```python
from build123d import *

# Parameters (mm, degrees)
SKETCH1_W           = 12.5
SKETCH1_H           = 4
SKETCH2_W           = 6
SKETCH2_H           = 2
SKETCH2_W_2         = 1.5
SKETCH2_H_2         = 1.5
SKETCH3_R           = 3.15
BOSS_EXTRUDE1_DEPTH = 1.3
SKETCH4_R           = 1.5
BOSS_EXTRUDE2_DEPTH = 4
CIRPATTERN1_COUNT   = 4
CHAMFER1_SIZE       = 1.3
CHAMFER1_SIZE_2     = 0.113735263


with BuildPart() as part:
    # Sketch1 → Revolve1 (revolve)
    with BuildSketch(Plane.XY, mode=Mode.PRIVATE) as revolve1_sk:
        with Locations((13.75, 2)):
            Rectangle(SKETCH1_W, SKETCH1_H)
    revolve(revolve1_sk.sketch.rotate(Axis((0, -5.176379432, 0), (0, 1, 0)), 90), axis=Axis((0, -5.176379432, 0), (0, 1, 0)))

    # Sketch2 → Cut-Revolve1 (revolve, cut)
    with BuildSketch(Plane.XY, mode=Mode.PRIVATE) as cut_revolve1_sk:
        with Locations((17, 1)):
            Rectangle(SKETCH2_W, SKETCH2_H)
        with Locations((8.25, 0.75)):
            Rectangle(SKETCH2_W_2, SKETCH2_H_2)
    revolve(cut_revolve1_sk.sketch.rotate(Axis((0, -1.233398275, 0), (0, 1, 0)), 90), axis=Axis((0, -1.233398275, 0), (0, 1, 0)), mode=Mode.SUBTRACT)

    # Sketch3 → Boss-Extrude1 (add)
    with BuildSketch(Plane(origin=(0, 4, 0), x_dir=(1, 0, 0), z_dir=(0, 1, 0))):
        with Locations(Location((17, 0, 0), (0, 0, 19.305796893))):
            Circle(SKETCH3_R)
    boss_extrude1 = extrude(amount=BOSS_EXTRUDE1_DEPTH)

    # Sketch4 → Boss-Extrude2 (add)
    with BuildSketch(Plane.XZ.offset(-2)):
        with Locations(Location((17, 0, 0), (0, 0, 90))):
            Circle(SKETCH4_R)
    boss_extrude2 = extrude(amount=BOSS_EXTRUDE2_DEPTH)

    # CirPattern1: Boss-Extrude1, Boss-Extrude2 ×4 about axis
    cirpattern1_axis = Axis((0, 0, 0), (0, 1, 0))
    add([boss_extrude1.rotate(cirpattern1_axis, i * 360 / CIRPATTERN1_COUNT) for i in range(1, CIRPATTERN1_COUNT)])
    add([boss_extrude2.rotate(cirpattern1_axis, i * 360 / CIRPATTERN1_COUNT) for i in range(1, CIRPATTERN1_COUNT)])

    # Chamfer1
    # the kernel refuses this chamfer: 1.3, 0.113735263 mm, written as the material it takes off along each edge
    with BuildSketch(Plane(origin=(17, 5.3, 0), x_dir=(0.9437675070022826, 0, -0.3306098799592901), z_dir=(0.3306098799592901, 0, 0.9437675070022826))) as chamfer1_piece_1_section:
        Polygon((3.15, -CHAMFER1_SIZE), (3.15 - CHAMFER1_SIZE_2 * 0.99999999634, 0), (3.15, 0), align=None)
    chamfer1_piece_1 = revolve(axis=Axis((17, 5.3, 0), (0, 1, 0)), mode=Mode.PRIVATE)
    chamfer1_piece_1 = split(chamfer1_piece_1, bisect_by=Plane(origin=(14.070685383, 4, 1.026164121), z_dir=(0, 1, 0)), keep=Keep.TOP, mode=Mode.PRIVATE)
    add(chamfer1_piece_1, mode=Mode.SUBTRACT)
    with BuildSketch(Plane(origin=(0, 5.3, 17), x_dir=(0.3306098799592899, 0, 0.9437675070022828), z_dir=(-0.9437675070022828, 0, 0.3306098799592899))) as chamfer1_piece_2_section:
        Polygon((3.15, -CHAMFER1_SIZE), (3.15 - CHAMFER1_SIZE_2 * 0.99999999634, 0), (3.15, 0), align=None)
    chamfer1_piece_2 = revolve(axis=Axis((0, 5.3, 17), (0, 1, 0)), mode=Mode.PRIVATE)
    chamfer1_piece_2 = split(chamfer1_piece_2, bisect_by=Plane(origin=(-1.026164121, 4, 14.070685383), z_dir=(0, 1, 0)), keep=Keep.TOP, mode=Mode.PRIVATE)
    add(chamfer1_piece_2, mode=Mode.SUBTRACT)
    with BuildSketch(Plane(origin=(-17, 5.3, 0), x_dir=(-0.9437675070022828, 0, 0.33060987995929), z_dir=(-0.33060987995929, 0, -0.9437675070022828))) as chamfer1_piece_3_section:
        Polygon((3.15, -CHAMFER1_SIZE), (3.15 - CHAMFER1_SIZE_2 * 0.99999999634, 0), (3.15, 0), align=None)
    chamfer1_piece_3 = revolve(axis=Axis((-17, 5.3, 0), (0, 1, 0)), mode=Mode.PRIVATE)
    chamfer1_piece_3 = split(chamfer1_piece_3, bisect_by=Plane(origin=(-14.070685383, 4, -1.026164121), z_dir=(0, 1, 0)), keep=Keep.TOP, mode=Mode.PRIVATE)
    add(chamfer1_piece_3, mode=Mode.SUBTRACT)
    with BuildSketch(Plane(origin=(0, 5.3, -17), x_dir=(-0.33060987995929003, 0, -0.9437675070022828), z_dir=(0.9437675070022828, 0, -0.33060987995929003))) as chamfer1_piece_4_section:
        Polygon((3.15, -CHAMFER1_SIZE), (3.15 - CHAMFER1_SIZE_2 * 0.99999999634, 0), (3.15, 0), align=None)
    chamfer1_piece_4 = revolve(axis=Axis((0, 5.3, -17), (0, 1, 0)), mode=Mode.PRIVATE)
    chamfer1_piece_4 = split(chamfer1_piece_4, bisect_by=Plane(origin=(1.026164121, 4, -14.070685383), z_dir=(0, 1, 0)), keep=Keep.TOP, mode=Mode.PRIVATE)
    add(chamfer1_piece_4, mode=Mode.SUBTRACT)


solid = part.part
```
Source: CAD feature listing. Evaluate the final solid. Frame: model axes, mm. A direction names the side the tool comes from. Coordinates: 2 decimals unless noted, no trailing zeros. Loops run counter-clockwise (first coordinate to the right, second up) from the corner with the lowest first, then second, coordinate; pieces in that order, holes last. Notation, with made-up numbers: M 13,46.25 L 37,46.25 A28 ccw 37,81.25 Z; hole C 14.5,88.25 d5. An arc over 180 degrees is marked long. Use a Markdown table: item, result. Add a question column.
Q1. Section query C-C, the plane y = -1.25. Return loops of the section in (x, z).
Q2. Section query D-D, the plane z = -6. Return loops of the section in (x, y).
Q3. Access query for faces 4 (the flat face through (9, 4, 0)), 5 (the flat face through (0, 5.3, -17)), 6 (the cylindrical face through (12.4, 1, -6.5)). Directions: +Z, -Z, +X, -X, +Y, -Y. A direction counts if a zero-diameter tool reaches every point of the face in a straight line with its end or side. Return the directions, or none.
Q4. Draft query along Z for faces 1 (the flat face through (-17, 5.3, 0)), 2 (the cylindrical face through (-15.513, 0.028, 0.195)), 3 (the cylindrical face through (-0.195, 0.028, -15.513)). Return one class per face: pulls with the +Z half, pulls with the -Z half, needs draft (parallel to the pull), parting line crosses it, or undercut.
Q5. Material intervals for L1, parallel to X at y = 0.95, z = 0; L2, parallel to Y at x = -8, z = -16; L3, parallel to X at y = 2.4, z = 0, sorted ascending.
Q6. First-contact query: pin 1 (24 mm diameter, centred on x = 0, z = 0, fed in from +Y); pin 2 (2 mm diameter, centred on x = -6.5, z = -11, fed in from -Y); pin 3 (4 mm diameter, centred on y = 1, z = -4.5, fed in from +X). Flat tips, straight axial feed; report the tip coordinate or a pass-through.
Result:
| question | item | result |
|---|---|---|
| 1 | outline | C -17,0 d3; C 0,-17 d3; C 0,17 d3; C 17,0 d3 |
| 2 | outline | M -19.08,2 L -12.65,2 L -12.65,0 L -6.71,0 L -6.71,1.5 L -4.5,1.5 L -4.5,4 L -19.08,4 Z; M 4.5,1.5 L 6.71,1.5 L 6.71,0 L 12.65,0 L 12.65,2 L 19.08,2 L 19.08,4 L 4.5,4 Z |
| 3 | face 4 | +Y |
| 3 | face 5 | +Z, -Z, +X, -X, +Y |
| 3 | face 6 | -Y |
| 4 | face 1 | needs draft |
| 4 | face 2 | parting line crosses it |
| 4 | face 3 | undercut |
| 5 | L1 | x = -18.5 to -15.5, -14 to -9, 9 to 14, 15.5 to 18.5 |
| 5 | L2 | y = 2 to 4 |
| 5 | L3 | x = -20 to -7.5, 7.5 to 20 |
| 6 | pin 1 | stops at y = 4 |
| 6 | pin 2 | stops at y = 0 |
| 6 | pin 3 | stops at x = 19.81 |
